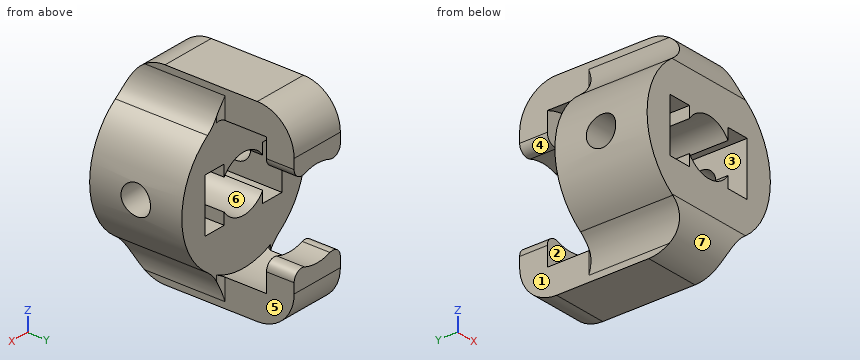
from build123d import *

# Parameters (mm, degrees)
SKETCH1_R               = 8
SKETCH1_R_2             = 3
BOSS_EXTRUDE1_DEPTH     = 10
BOSS_EXTRUDE2_DEPTH     = 15
BOSS_EXTRUDE3_DEPTH     = 3
FILLET1_R               = 4
FILLET2_R               = 4
FILLET3_R               = 0.5
FILLET4_R               = 1
CUT_EXTRUDE1_DEPTH      = 56.872699751
CUT_EXTRUDE1_DEPTH_BACK = 56.872699751
SKETCH5_R               = 1.6
CUT_EXTRUDE2_REACH      = 55.831
SKETCH6_W               = 2.5
SKETCH6_H               = 5.8


with BuildPart() as part:
    # Sketch1 → Boss-Extrude1 (new body)
    with BuildSketch(Plane(origin=(0, 0, 0), x_dir=(1, 0, 0), z_dir=(0, 1, 0))):
        with Locations(Location((-42.590141196, -5.023885001, 0), (0, 0, 270))):
            Circle(SKETCH1_R)
        with Locations(Location((-42.590141196, -5.023885001, 0), (0, 0, 270))):
            Circle(SKETCH1_R_2, mode=Mode.SUBTRACT)
    extrude(amount=BOSS_EXTRUDE1_DEPTH)

    # Sketch2 → Boss-Extrude2 (add)
    with BuildSketch(Plane(origin=(0, 0, 0), x_dir=(1, 0, 0), z_dir=(0, 1, 0))):
        with BuildLine():
            Line((-39.590141196, -12.440083488), (-39.590141196, -15.440083488))
            Line((-39.590141196, -15.440083488), (-45.590141196, -15.440083488))
            Line((-45.590141196, -15.440083488), (-45.590141196, -12.440083488))
            ThreePointArc((-45.590141196, -12.440083488), (-42.590141196, -13.023885001), (-39.590141196, -12.440083488))
        make_face()
        with BuildLine():
            Line((-45.590141196, 5.392313486), (-45.590141196, 2.392313486))
            ThreePointArc((-45.590141196, 2.392313486), (-42.590141196, 2.976114999), (-39.590141196, 2.392313486))
            Line((-39.590141196, 2.392313486), (-39.590141196, 5.392313486))
            Line((-39.590141196, 5.392313486), (-45.590141196, 5.392313486))
        make_face()
    extrude(amount=BOSS_EXTRUDE2_DEPTH)

    # Sketch3 → Boss-Extrude3 (add)
    with BuildSketch(Plane(origin=(0, 15, 0), x_dir=(1, 0, 0), z_dir=(0, 1, 0))):
        with BuildLine():
            Line((-39.590141196, -15.440083488), (-45.590141196, -15.440083488))
            Line((-45.590141196, -15.440083488), (-45.590141196, -8.660434161))
            ThreePointArc((-45.590141196, -8.660434161), (-42.590141196, -9.738170715), (-39.590141196, -8.660434161))
            Line((-39.590141196, -8.660434161), (-39.590141196, -15.440083488))
        make_face()
        with BuildLine():
            Line((-45.590141196, 5.392313486), (-45.590141196, -1.38733584))
            ThreePointArc((-45.590141196, -1.38733584), (-42.590141196, -0.309599286), (-39.590141196, -1.38733584))
            Line((-39.590141196, -1.38733584), (-39.590141196, 5.392313486))
            Line((-39.590141196, 5.392313486), (-45.590141196, 5.392313486))
        make_face()
    extrude(amount=BOSS_EXTRUDE3_DEPTH)

    # Fillet1
    fillet1_edges = [part.edges().sort_by_distance(p)[0] for p in [
        (-39.590141196, 5, 12.440083488),
        (-45.590141196, 5, 12.440083488),
        (-45.590141196, 5, -2.392313486),
        (-39.590141196, 5, -2.392313486),
    ]]
    fillet(fillet1_edges, radius=FILLET1_R)

    # Fillet2
    fillet2_edges = [part.edges().sort_by_distance(p)[0] for p in [
        (-42.590141196, 18, 15.440083488),
        (-42.590141196, 18, -5.392313486),
        (-42.590141196, 0, -5.392313486),
        (-42.590141196, 0, 15.440083488),
    ]]
    fillet(fillet2_edges, radius=FILLET2_R)

    # Fillet3
    fillet3_edges = [part.edges().sort_by_distance(p)[0] for p in [
        (-39.590141196, 10, -3.557611415),
        (-39.590141196, 10, 13.605381417),
        (-45.590141196, 10, 13.605381417),
        (-45.590141196, 10, -3.557611415),
    ]]
    fillet(fillet3_edges, radius=FILLET3_R)

    # Fillet4
    fillet4_edges = [part.edges().sort_by_distance(p)[0] for p in [
        (-39.590141196, 16.5, 8.660434161),
        (-45.590141196, 16.5, 8.660434161),
        (-45.590141196, 16.5, 1.38733584),
        (-39.590141196, 16.5, 1.38733584),
    ]]
    fillet(fillet4_edges, radius=FILLET4_R)

    # Sketch5 → Cut-Extrude1 (cut, two sides: drawn at the far end of the back side and taken through both)
    with BuildSketch(Plane(origin=(0, 0, 0), x_dir=(0, 0, -1), z_dir=(1, 0, 0)).offset(-CUT_EXTRUDE1_DEPTH_BACK)):
        with Locations((-5.023885001, 5)):
            Circle(SKETCH5_R)
    extrude(amount=CUT_EXTRUDE1_DEPTH + CUT_EXTRUDE1_DEPTH_BACK, mode=Mode.SUBTRACT)

    # Sketch6 → Cut-Extrude2 (cut, up to next)
    with BuildSketch(Plane(origin=(0, 10, 0), x_dir=(1, 0, 0), z_dir=(0, 1, 0)), mode=Mode.PRIVATE) as cut_extrude2_sk1:
        with Locations((-38.840141196, -5.023885001)):
            Rectangle(SKETCH6_W, SKETCH6_H)
    cut_extrude2_tool1 = extrude(cut_extrude2_sk1.sketch, amount=-CUT_EXTRUDE2_REACH, mode=Mode.PRIVATE) & part.part
    # Sketch6 → Cut-Extrude2 (cut, up to next)
    with BuildSketch(Plane(origin=(0, 10, 0), x_dir=(1, 0, 0), z_dir=(0, 1, 0)), mode=Mode.PRIVATE) as cut_extrude2_sk2:
        with Locations((-46.340141196, -5.023885001)):
            Rectangle(SKETCH6_W, SKETCH6_H)
    cut_extrude2_tool2 = extrude(cut_extrude2_sk2.sketch, amount=-CUT_EXTRUDE2_REACH, mode=Mode.PRIVATE) & part.part
    add(cut_extrude2_tool1.solids().sort_by_distance((-38.840141, 10, 5.023885))[0], mode=Mode.SUBTRACT)
    add(cut_extrude2_tool2.solids().sort_by_distance((-46.340141, 10, 5.023885))[0], mode=Mode.SUBTRACT)


solid = part.part
The listing builds one solid part. Answer for the finished solid, in the listing's coordinates (mm). Face numbers are marked on the shaded views. A direction names the side the tool comes from. Round coordinates to 2 decimals unless told otherwise and drop trailing zeros. Loops run counter-clockwise (first coordinate to the right, second up) from the corner with the lowest first, then second, coordinate; pieces in that order, holes last. Notation, with made-up numbers: M 85.25,16.25 L 107.25,16.25 A24 cw 107.25,44.25 Z; hole C -39.75,-30 d4. An arc over 180 degrees is marked long. Return JSON: item names as keys, results as strings.
Q1. Each of these flat-tipped pins is pushed along its axis until it touches: pin 1 Ø5 at (y, z) = (2.5, 3) entering from +X; pin 2 Ø4 at (y, z) = (7, 13.5) entering from +X; pin 3 Ø1.5 at (y, z) = (2.5, 12.5) entering from -X; pin 4 Ø0.6 at (y, z) = (3.5, 3) entering from -X. Where does it stop, or does it pass through?
Results list:
{"pin 1": "stops at x = -34.59", "pin 2": "stops at x = -37.89", "pin 3": "stops at x = -46.97", "pin 4": "stops at x = -50.4"}
Q2. Find the intervals of material crossed by line 1 along Y through (x, z) = (-42.5, 12.5); line 2 along X through (y, z) = (1.5, 5); line 3 along Z through (x, y) = (-49.8, 5), in increasing order. Write a range as from..to.
Results list:
{"line 1": "y = 0.14..10, 15..17.86", "line 2": "x = -50.59..-47.59, -37.59..-34.59", "line 3": "z = 1.56..3.42, 6.62..8.49"}
Q3. Find section D-D, the plane z = 10.75. Determine the outline of the cut face in (x, y), plus the area to 3 significant figures.
Results list:
{"outline": "M -48.18,0 L -37,0 L -37,10 L -48.18,10 Z; M -45.59,15 L -39.59,15 L -39.59,18 L -45.59,18 Z", "area": "130 mm2"}
Q4. The mould has two halves that part along Z. Classify the marked faces 5, 6 and 7: released by +Z, released by -Z, zero draft, split by the parting line, or undercut.
Results list:
{"face 5": "zero draft", "face 6": "undercut", "face 7": "released by -Z"}
Q5. Find section B-B, the plane y = 9.5. Determine the outline of the cut face in (x, z), plus the area to 3 significant figures.
Results list:
{"outline": "M -47.26,-1.47 A4 cw -45.59,-4.72 L -45.59,-5.39 L -39.59,-5.39 L -39.59,-4.72 A4 cw -37.92,-1.47 A8 ccw -37.92,11.52 A4 cw -39.59,14.77 L -39.59,15.44 L -45.59,15.44 L -45.59,14.77 A4 cw -47.26,11.52 A8 ccw Z; hole M -47.59,2.12 L -45.09,2.12 L -45.09,3.37 A3 ccw -40.09,3.37 L -40.09,2.12 L -37.59,2.12 L -37.59,7.92 L -40.09,7.92 L -40.09,6.68 A3 ccw -45.09,6.68 L -45.09,7.92 L -47.59,7.92 Z", "area": "180 mm2"}
Q6. Find section C-C, the plane x = -44.5. Determine the outline of the cut face in (y, z).
Results list:
{"outline": "M 0,-1.39 A4 ccw 4,-5.39 L 14,-5.39 A4 ccw 18,-1.39 L 18,0.67 L 15,0.67 L 15,-2.74 L 10,-2.74 L 10,2.71 L 0,2.71 Z; M 0,7.34 L 10,7.34 L 10,12.79 L 15,12.79 L 15,9.38 L 18,9.38 L 18,11.44 A4 ccw 14,15.44 L 4,15.44 A4 ccw 0,11.44 Z"}
Q7. Find section A-A, the plane z = 4.5. Determine the outline of the cut face in (x, y), plus the area to 3 significant figures.
Results list:
{"outline": "M -50.57,0 L -47.59,0 L -47.59,3.49 L -50.57,3.49 Z; M -50.57,6.51 L -47.59,6.51 L -47.59,10 L -50.57,10 Z; M -37.59,0 L -34.61,0 L -34.61,3.49 L -37.59,3.49 Z; M -37.59,6.51 L -34.61,6.51 L -34.61,10 L -37.59,10 Z", "area": "41.6 mm2"}
Q8. Which of the six approach directions +Z, -Z, +X, -X, +Y, -Y give full straight-line access (tool end or side, diameter ignored) to the marked faces 1, 2, 3 and 4?
Results list:
{"face 1": "-Z, -X, +Y", "face 2": "none", "face 3": "+Y, -Y", "face 4": "+Y"}
